Here's the drawing with two shaded views (mm, measured from the low corner). I have some questions. A direction names the side the tool comes from. Round coordinates to 2 decimals unless told otherwise and drop trailing zeros. Loops run counter-clockwise (first coordinate to the right, second up) from the corner with the lowest first, then second, coordinate; pieces in that order, holes last. Notation, with made-up numbers: (-24.75, 17.25) -> (19.25, 17.25) arc R6 cw to (19.25, 22.25) -> close; hole circle Ø1 at (44.5, 74). An arc over 180 degrees is marked (long way). Use a Markdown table: item, result.
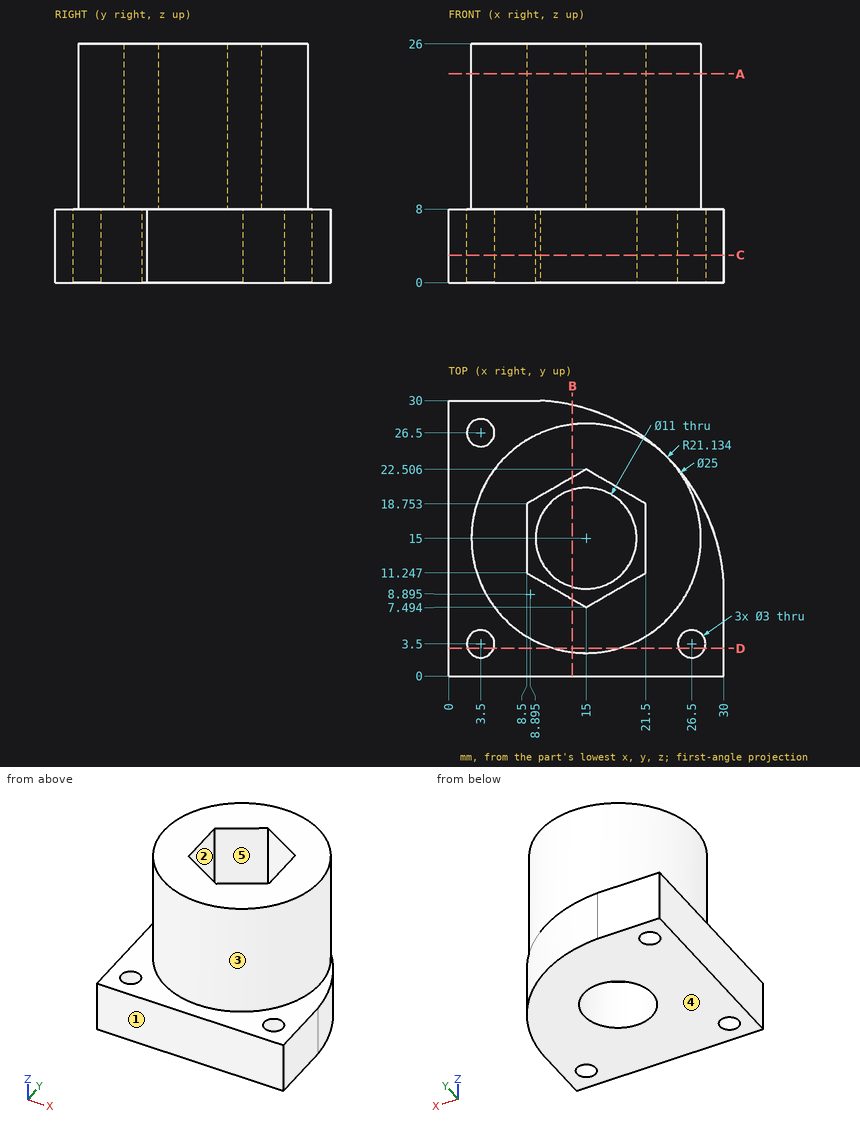
1. Which directions (+Z, -Z, +X, -X, +Y, -Y) give clear straight access to the entire face, cutting with the end or side of a thin tool? Please do the marked faces 4 and 5.
Answer sheet:
| item | result |
|---|---|
| face 4 | -Z, +X, -X, +Y, -Y |
| face 5 | +Z |
2. I want a section at B-B (x = 13.5). Please give me the cut outline in (y, z), plus the area to 3 significant figures.
Answer sheet:
| item | result |
|---|---|
| outline | (0, 0) -> (9.71, 0) -> (9.71, 8) -> (8.36, 8) -> (8.36, 26) -> (2.59, 26) -> (2.59, 8) -> (0, 8) -> close; (20.29, 0) -> (29.52, 0) -> (29.52, 8) -> (27.41, 8) -> (27.41, 26) -> (21.64, 26) -> (21.64, 8) -> (20.29, 8) -> close |
| area | 359 mm² |
3. I need wall thicknesses on line 1 (Y direction, x = 3.5, z = 5.5); line 2 (Y direction, x = 14.75, z = 1.5) (1 decimal); line 3 (X direction, y = 20, z = 3.75) (1 decimal). Which ranges of each line are inside material? Lowest first, please.
Answer sheet:
| item | result |
|---|---|
| line 1 | y = 0 to 2, 5 to 25, 28 to 30 |
| line 2 | y = 0 to 9.5, 20.5 to 29.2 |
| line 3 | x = 0 to 12.7, 17.3 to 26.9 |
4. I want a section at A-A (z = 22.75). Please give me the cut outline in (x, y) (1 decimal).
Answer sheet:
| item | result |
|---|---|
| outline | circle Ø25 at (15, 15); hole (8.5, 11.2) -> (15, 7.5) -> (21.5, 11.2) -> (21.5, 18.8) -> (15, 22.5) -> (8.5, 18.8) -> close |
5. Will these pins go through, and if not, where does the flat tip stop? pin 1 Ø4 at (x, y) = (3.5, 26.5) entering from +Z; pin 2 Ø10 at (y, z) = (25, 15) entering from -X; pin 3 Ø2 at (y, z) = (24, 13) entering from +X (1 decimal).
Answer sheet:
| item | result |
|---|---|
| pin 1 | stops at z = 8 |
| pin 2 | stops at x = 3.54 |
| pin 3 | stops at x = 24.6 |
6. I want a section at D-D (y = 3). Please give me the cut outline in (x, z) (1 decimal), plus the area to 3 significant figures.
Answer sheet:
| item | result |
|---|---|
| outline | (0, 0) -> (2.1, 0) -> (2.1, 8) -> (0, 8) -> close; (4.9, 0) -> (25.1, 0) -> (25.1, 8) -> (18.5, 8) -> (18.5, 26) -> (11.5, 26) -> (11.5, 8) -> (4.9, 8) -> close; (27.9, 0) -> (30, 0) -> (30, 8) -> (27.9, 8) -> close |
| area | 321 mm² |
7. I want a section at C-C (z = 3). Please give me the cut outline in (x, y) (1 decimal), plus the area to 3 significant figures.
Answer sheet:
| item | result |
|---|---|
| outline | (0, 0) -> (30, 0) -> (30, 10) arc R21.1 ccw to (10, 30) -> (0, 30) -> close; hole circle Ø3 at (3.5, 3.5); hole circle Ø3 at (3.5, 26.5); hole circle Ø11 at (15, 15); hole circle Ø3 at (26.5, 3.5) |
| area | 689 mm² |
8. If we mould it in two halves opening along X, with no side actions, what happens to the marked faces 1, 2 and 3? For each: +X half, -X half, draft (parallel to the pull), parting line (faces both ways), or undercut.
Answer sheet:
| item | result |
|---|---|
| face 1 | draft |
| face 2 | undercut |
| face 3 | parting line |
